Design review of the part shown in the three views and the two pictorial views. Dimensions are in mm from the part's minimum x, y and z. A direction names the side the tool comes from. Round coordinates to 2 decimals unless told otherwise and drop trailing zeros. Loops run counter-clockwise (first coordinate to the right, second up) from the corner with the lowest first, then second, coordinate; pieces in that order, holes last. Notation, with made-up numbers: (49.5, 3.5) -> (79.5, 3.5) arc R6 cw to (79.5, 14.5) -> close; hole circle Ø2 at (84, 66). An arc over 180 degrees is marked (long way). Use a Markdown table: item, result. Add a question column.
1) Wall thickness on probe 1 along Y at (x, z) = (34.5, 18); probe 2 along Z at (x, y) = (52, 26); probe 3 along Y at (x, z) = (53.5, 15.5): over which ranges is each line inside the solid? List them lowest first.
2) Consider section A-A on y = 35. Give the boundary of the cut face in (x, z), plus the area to 3 significant figures.
3) Consider section B-B on x = 21. Give the boundary of the cut face in (y, z).
4) Consider section D-D on x = 37. Give the boundary of the cut face in (y, z), plus the area to 3 significant figures.
5) Insertion check: pin 1 (12 mm diameter, centred on x = 55.5, y = 33, fed in from -Z); pin 2 (7.5 mm diameter, centred on y = 11, z = 29.5, fed in from -X); pin 3 (1 mm diameter, centred on y = 45, z = 38, fed in from -X). Each pin has a flat end and moves straight along its axis. Give the tip position at first contact, or say it passes through.
6) Mouldability with a two-part tool opening along Y and no side actions: class the marked faces 4, 5 and 6 as released by +Y, released by -Y, zero draft, split by the parting line, or undercut.
7) Consider section C-C on z = 33. Give the boundary of the cut face in (x, y), plus the area to 4 significant figures.
8) For the marked faces 1, 2 and 3, list the 3-axis set-ups (+Z, -Z, +X, -X, +Y, -Y) from which the entire face can be reached by the end or side of a thin tool; tool diameter is ignored.
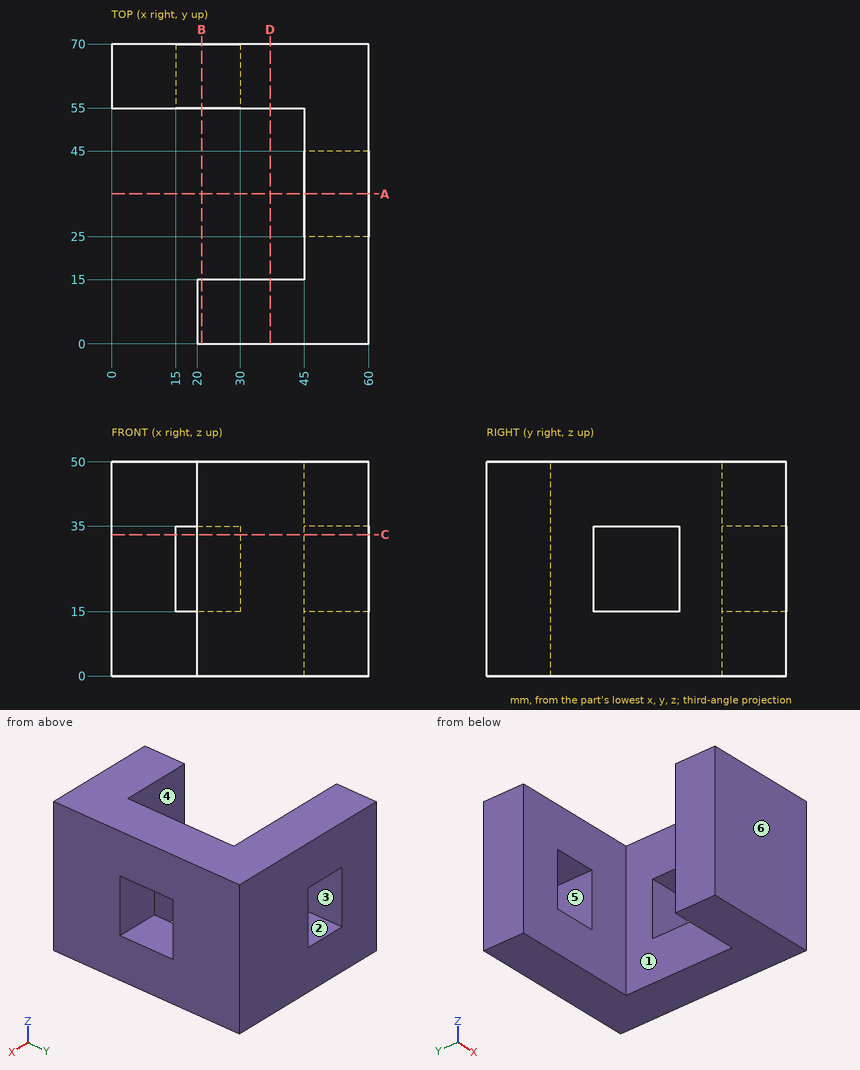
Result set:
| question | item | result |
|---|---|---|
| 1 | probe 1 | 0 to 15, 55 to 70 |
| 1 | probe 2 | 0 to 15, 35 to 50 |
| 1 | probe 3 | 0 to 25, 45 to 70 |
| 2 | outline | (45, 0) -> (60, 0) -> (60, 15) -> (45, 15) -> close; (45, 35) -> (60, 35) -> (60, 50) -> (45, 50) -> close |
| 2 | area | 450 mm2 |
| 3 | outline | (0, 0) -> (15, 0) -> (15, 50) -> (0, 50) -> close; (55, 0) -> (70, 0) -> (70, 15) -> (55, 15) -> close; (55, 35) -> (70, 35) -> (70, 50) -> (55, 50) -> close |
| 4 | outline | (0, 0) -> (15, 0) -> (15, 50) -> (0, 50) -> close; (55, 0) -> (70, 0) -> (70, 50) -> (55, 50) -> close |
| 4 | area | 1,500 mm2 |
| 5 | pin 1 | z = 0 |
| 5 | pin 2 | x = 20 |
| 5 | pin 3 | x = 45 |
| 6 | face 4 | undercut |
| 6 | face 5 | zero draft |
| 6 | face 6 | released by -Y |
| 7 | outline | (0, 55) -> (15, 55) -> (15, 70) -> (0, 70) -> close; (20, 0) -> (60, 0) -> (60, 25) -> (45, 25) -> (45, 15) -> (20, 15) -> close; (30, 55) -> (45, 55) -> (45, 45) -> (60, 45) -> (60, 70) -> (30, 70) -> close |
| 7 | area | 1,575 mm2 |
| 8 | face 1 | +Z, -Z, -X |
| 8 | face 2 | +Y |
| 8 | face 3 | +Y, -Y |
